Read the model definition and answer for the solid it produces. Units are mm, in the model's axes. Face numbers are marked on the shaded views. A direction names the side the tool comes from. Give positions to 0.01 mm unless a question says otherwise; leave off trailing zeros. Loops run counter-clockwise (first coordinate to the right, second up) from the corner with the lowest first, then second, coordinate; pieces in that order, holes last. Notation, with made-up numbers: (-34.75, 78) -> (0.25, 78) arc R11 ccw to (0.25, 87) -> close; hole circle Ø2 at (36, 2). An arc over 180 degrees is marked (long way). Write each question's results on one line, items separated by ' | '. Start each with the question number.
Item 1: Each of these flat-tipped pins is pushed along its axis until it touches: P1, Ø6, axis at x = 52, z = 8.5, coming from the +Y side; P2, Ø4, axis at x = 53.89, y = -33.99, coming from the +Z side; P3, Ø4, axis at x = 55, y = -35, coming from the -Z side. Where does it stop, or does it pass through?
Item 2: Find the intervals of material crossed by line 1 (X direction, y = -5.5, z = 12); line 2 (Y direction, x = 23, z = 5); line 3 (Z direction, x = 51.5, y = -36), in increasing order.
Item 3: Which of the six approach directions +Z, -Z, +X, -X, +Y, -Y give full straight-line access (tool end or side, diameter ignored) to the marked faces 1, 2 and 3?
Item 4: Section D-D on y = -35 is taken. State how many separate pieces and enclosed holes the cut face has, and give its area (3 significant figures).
Item 5: Section B-B on y = -19 is taken. Write down the section's boundary in (x, z), and give its area (3 significant figures).
Item 6: Section C-C on x = -2 is taken. Write down the section's boundary in (y, z), and give its area (3 significant figures).
Item 7: Section A-A on z = 1 is taken. Write down the section's boundary in (x, y).
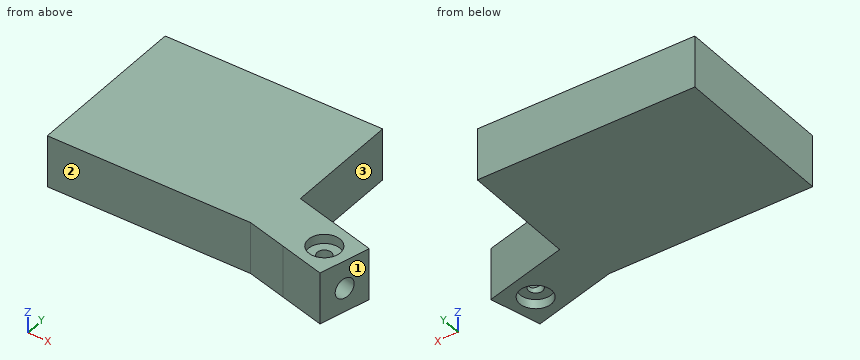
```python
from build123d import *

# Parameters (mm, degrees)
F0_R     = 1.7272
F1_DEPTH = 12.7
F2_R     = 2.4511
F3_DEPTH = 16.51
F4_R     = 3.8989
F4_R_2   = 1.7272
F5_DEPTH = 2.286
F6_R     = 3.8989
F6_R_2   = 1.7272
F7_DEPTH = 2.286


with BuildPart() as f1:
    # F0 (on Top) → F1 (new body)
    with BuildSketch(Plane.XY):
        Polygon((40.905171, 4.372339), (-12.235096, 4.372339), (-12.235096, -11.662856), (-12.235096, -36.157189), (-1.651831, -36.157189), (37.463617, -36.157189), (47.219385, -38.77124), (58.382782, -41.762463), (61.669784, -29.495205), (40.905171, -23.931344), (40.905171, -11.662856), align=None)
        with Locations((53.892654, -33.985333)):
            Circle(F0_R, mode=Mode.SUBTRACT)
    extrude(amount=F1_DEPTH)

    # F2 (on face) → F3 (cut)
    with BuildSketch(Plane(origin=(64.912493, -17.39325, 0), x_dir=(0.258819, 0.965926, 0), z_dir=(0.965926, -0.258819, 0))):
        with Locations((-18.878866, 5.865277)):
            Circle(F2_R)
    extrude(amount=-F3_DEPTH, mode=Mode.SUBTRACT)

    # F4 (on face) → F5 (cut)
    with BuildSketch(Plane.XY.offset(12.7)):
        with Locations((53.892654, -33.985333)):
            Circle(F4_R)
        with Locations((53.892654, -33.985333)):
            Circle(F4_R_2, mode=Mode.SUBTRACT)
    extrude(amount=-F5_DEPTH, mode=Mode.SUBTRACT)

    # F6 (on face) → F7 (cut)
    with BuildSketch(Plane(origin=(0, 0, 0), x_dir=(1, 0, 0), z_dir=(0, 0, -1))):
        with Locations((53.892654, 33.985333)):
            Circle(F6_R)
        with Locations((53.892654, 33.985333)):
            Circle(F6_R_2, mode=Mode.SUBTRACT)
    extrude(amount=-F7_DEPTH, mode=Mode.SUBTRACT)


solid = f1.part
```
Findings:
1) P1: y = -26.1 | P2: z = 10.41 | P3: z = 2.29
2) line 1: -12.24 to 40.91 | line 2: -36.16 to 4.37 | line 3: 2.29 to 10.41
3) face 1: +Z, -Z, +X, -Y | face 2: +Z, -Z, -X, -Y | face 3: +Z, -Z, +X, +Y
4) separate pieces: 3 | enclosed holes: 0 | area: 827 mm2
5) outline: (-12.24, 0) -> (40.91, 0) -> (40.91, 12.7) -> (-12.24, 12.7) -> close | area: 675 mm2
6) outline: (-36.16, 0) -> (4.37, 0) -> (4.37, 12.7) -> (-36.16, 12.7) -> close | area: 515 mm2
7) outline: (-12.24, -36.16) -> (37.46, -36.16) -> (58.38, -41.76) -> (61.67, -29.5) -> (40.91, -23.93) -> (40.91, 4.37) -> (-12.24, 4.37) -> close; hole circle Ø7.8 at (53.89, -33.99)
